Source: CAD feature listing. Evaluate the final solid. Frame: model axes, mm. A direction names the side the tool comes from. Round coordinates to 2 decimals unless told otherwise and drop trailing zeros. Order: outer loops, then holes, each group sorted by start corner. A loop starts at its lowest first (then second) coordinate and runs counter-clockwise, first axis right, second up. Notation, with made-up numbers: (45.5, 17.25) -> (55.5, 17.25) arc R21 cw to (55.5, 30.25) -> close; hole circle Ø6 at (-8, -21.5). An arc over 180 degrees is marked (long way). Answer as CSV lines item,"result". Start each with the question number.
(1) Contact query for flat-ended pins moving along their axis: P1, Ø0.8, axis at x = -31, z = -23.5, coming from the +Y side; P2, Ø3, axis at x = -8.5, z = -44.5, coming from the +Y side. Output: stop coordinate, or through.
(2) Section query D-D (x = -21.5). Output: boundary loops of the cut face in (y, z), plus the area to 3 significant figures.
(3) Pull-direction query (Z, two-part tool) for faces 3 (the flat face through (-31, 7, 0)), 4 (the flat face through (-16.25, 4, -29)), 5 (the flat face through (-31, 15, -1)); classes: +Z half, -Z half, draft (parallel to the pull), parting line (faces both ways), or undercut.
(4) Set-up query: faces 1 (the flat face through (-31, 0, -29)), 2 (the flat face through (-54, 1, -29)). Return all of +Z, -Z, +X, -X, +Y, -Y with unobstructed straight access to the full face (end or side cutting, diameter ignored); none if empty.
(5) Section query B-B (y = 2). Output: boundary loops of the cut face in (x, z), plus the area to 4 significant figures.
(6) Line query: line 1 along X through (y, z) = (4.5, -41); line 2 along Z through (x, y) = (-48, 3.5); line 3 along X through (y, z) = (7.25, -41.5). Output: solid intervals per line, ascending. Write a range as from..to.
(7) Section query A-A (y = 7.5). Output: boundary loops of the cut face in (x, z), plus the area to 3 significant figures.
(8) Section query C-C (z = -3.5). Output: boundary loops of the cut face in (x, y), plus the area to 3 significant figures.
Autodesk Inventor part; units mm, degrees
ref_plane "YZ Plane" through (0, 0, 0) normal (1, 0, 0) x (0, 1, 0)
ref_plane "XZ Plane" through (0, 0, 0) normal (0, 1, 0) x (-1, 0, 0)
ref_plane "XY Plane" through (0, 0, 0) normal (0, 0, 1) x (1, 0, 0)
sketch "Sketch1" plane through (0, 0, 0) normal (0, 1, 0) x (-1, 0, 0)
  line L0 (0, 0) -> (62, 0)
  line L1 (62, 0) -> (62, -58)
  line L2 (62, -58) -> (0, -58)
  line L3 (0, -58) -> (0, 0)
  dimension "d0" = 62
  dimension "d1" = 58
extrude "Extrusion1" add sketch "Sketch1" along normal blind 15
sketch "Sketch2" plane through (0, 0, -58) normal (0, 0, -1) x (-1, 0, 0)
  line L0 (62, 0) -> (0, 0)
  line L1 (0, 0) -> (62, 0)
  line L2 (62, 0) -> (62, 10)
  line L3 (57, 15) -> (5, 15)
  line L4 (0, 10) -> (0, 0)
  arc A0 (5, 15) -> (0, 10) centre (5, 10) ccw
  arc A1 (62, 10) -> (57, 15) centre (57, 10) ccw
  line L5 (0, 10) -> (-2.4331, 10)
  line L6 (-2.4331, 10) -> (-2.4331, 19.594)
  line L7 (-2.4331, 19.594) -> (72.365, 19.594)
  line L8 (72.365, 19.594) -> (72.365, 10)
  line L9 (72.365, 10) -> (62, 10)
  point P0 (62, 15)
  dimension "d4" = 5
extrude "Extrusion2" cut sketch "Sketch2" against normal up to surface (58 mm away) contours A1 L3 A0 L5 L6 L7 L8 L9
sketch "Sketch3" plane through (0, 15, 0) normal (0, 1, 0) x (1, 0, 0)
  line L0 (-1, 2.25) -> (-61, 2.25)
  line L1 (-61, 2.25) -> (-61, 55.75)
  line L2 (-61, 55.75) -> (-1, 55.75)
  line L3 (-1, 55.75) -> (-1, 2.25)
  line L4 (-57, 0) -> (-5, 0)
  line L5 (-5, 58) -> (-57, 58)
  line L6 (-62, 0) -> (-62, 58)
  line L7 (0, 58) -> (0, 0)
  dimension "d7" = 2.25
  dimension "d8" = 2.25
  dimension "d9" = 1
  dimension "d10" = 1
extrude "Extrusion3" cut sketch "Sketch3" against normal blind 14
sketch "Sketch4" plane through (0, 1, 0) normal (0, 1, 0) x (1, 0, 0)
  line L0 (-5, 2.25) -> (-57, 2.25)
  line L1 (-57, 55.75) -> (-5, 55.75)
  line L2 (-15.25, 2.25) -> (-16.25, 2.25)
  line L3 (-16.25, 2.25) -> (-16.25, 55.75)
  line L4 (-16.25, 55.75) -> (-15.25, 55.75)
  line L5 (-15.25, 55.75) -> (-15.25, 2.25)
  line L6 (-30.5, 2.25) -> (-31.5, 2.25)
  line L7 (-31.5, 2.25) -> (-31.5, 55.75)
  line L8 (-31.5, 55.75) -> (-30.5, 55.75)
  line L9 (-30.5, 55.75) -> (-30.5, 2.25)
  line L10 (-45.75, 2.25) -> (-46.75, 2.25)
  line L11 (-46.75, 2.25) -> (-46.75, 55.75)
  line L12 (-46.75, 55.75) -> (-45.75, 55.75)
  line L13 (-45.75, 55.75) -> (-45.75, 2.25)
  line L14 (-61, 2.25) -> (-61, 55.75)
  line L15 (-1, 55.75) -> (-1, 2.25)
  point P0 (0, 0)
  dimension "d13" = 1
  dimension "d14" = 1
  dimension "d15" = 1
  dimension "d16" = 14.25
  dimension "d17" = 14.25
  dimension "d18" = 14.25
extrude "Extrusion4" add sketch "Sketch4" along normal blind 5.25 contours L0 L3 L1 L5 | L0 L7 L1 L9 | L0 L11 L1 L13
properties part number "RoughBatteryPack"
Answer block:
1,P1,"y = 6.25"
1,P2,"y = 1"
2,outline,"(0, -58) -> (15, -58) -> (15, -55.75) -> (1, -55.75) -> (1, -2.25) -> (15, -2.25) -> (15, 0) -> (0, 0) -> close"
2,area,"121 mm2"
3,face 3,"+Z half"
3,face 4,"undercut"
3,face 5,"draft"
4,face 1,"+Z, -Z, +X, -X, -Y"
4,face 2,"+Y"
5,outline,"(-62, -58) -> (0, -58) -> (0, 0) -> (-62, 0) -> close; hole (-61, -55.75) -> (-46.75, -55.75) -> (-46.75, -2.25) -> (-61, -2.25) -> close; hole (-45.75, -55.75) -> (-31.5, -55.75) -> (-31.5, -2.25) -> (-45.75, -2.25) -> close; hole (-30.5, -55.75) -> (-16.25, -55.75) -> (-16.25, -2.25) -> (-30.5, -2.25) -> close; hole (-15.25, -55.75) -> (-1, -55.75) -> (-1, -2.25) -> (-15.25, -2.25) -> close"
5,area,"546.5 mm2"
6,line 1,"-62..-61, -46.75..-45.75, -31.5..-30.5, -16.25..-15.25, -1..0"
6,line 2,"-58..-55.75, -2.25..0"
6,line 3,"-62..-61, -1..0"
7,outline,"(-62, -58) -> (0, -58) -> (0, 0) -> (-62, 0) -> close; hole (-61, -55.75) -> (-1, -55.75) -> (-1, -2.25) -> (-61, -2.25) -> close"
7,area,"386 mm2"
8,outline,"(-62, 0) -> (0, 0) -> (0, 10) arc R5 ccw to (-1, 13) -> (-1, 1) -> (-15.25, 1) -> (-15.25, 6.25) -> (-16.25, 6.25) -> (-16.25, 1) -> (-30.5, 1) -> (-30.5, 6.25) -> (-31.5, 6.25) -> (-31.5, 1) -> (-45.75, 1) -> (-45.75, 6.25) -> (-46.75, 6.25) -> (-46.75, 1) -> (-61, 1) -> (-61, 13) arc R5 ccw to (-62, 10) -> close"
8,area,"99.8 mm2"
